```python
from build123d import *

# Parameters (mm, degrees)
F0_R     = 1.5
F1_DEPTH = 10
F2_DEPTH = 5
F3_DEPTH = 3


with BuildPart() as f1:
    # F0 (on Top) → F1 (new body)
    with BuildSketch(Plane.XY):
        Circle(F0_R)
    extrude(amount=F1_DEPTH)

    # F0 (on Top) → F2 (join)
    with BuildSketch(Plane.XY):
        Polygon((1.31021, 2.26935), (-1.31021, 2.26935), (-2.62042, 0), (-1.31021, -2.26935), (1.31021, -2.26935), (2.62042, 0), align=None)
        Circle(F0_R, mode=Mode.SUBTRACT)
    extrude(amount=F2_DEPTH)

    # F0 (on Top) → F3 (cut)
    with BuildSketch(Plane.XY):
        Circle(F0_R)
    extrude(amount=F3_DEPTH, mode=Mode.SUBTRACT)


solid = f1.part
```
For this review, take the finished solid that the model builds, in its own axes (mm). A direction names the side the tool comes from. Give positions to 0.01 mm unless a question says otherwise; leave off trailing zeros. Write each loop counter-clockwise with the first axis right and the second up, starting at its lowest first coordinate (ties: lowest second). Pieces come first, ordered by that corner, then holes.
Item 1: The part is to be moulded in two halves that separate along Y. For faces 3 (the face through (0, 2, 0)), 4 (the face through (0, 0, 3)), 5 (the face through (1.974, 1.119, 2.465)), 6 (the face through (-1.5, 0.07, 1.48)), say which applies: +Y half, -Y half, draft (parallel to the pull), parting line (faces both ways), or undercut.
Item 2: Wall thickness on probe 1 along Y at (x, z) = (0, 1.45); probe 2 along Z at (x, y) = (-0.5, 0.45); probe 3 along X at (y, z) = (-0.55, 2.5): over which ranges is each line inside the solid? List them lowest first.
Item 3: Take a section at B-B (x = 0). Give the boundary of the cut face in (y, z), and give its area (3 significant figures).
Item 4: Take a section at D-D (y = 0.15). Give the boundary of the cut face in (x, z), and give its area (3 significant figures).
Item 5: Take a section at A-A (z = 2). Give the boundary of the cut face in (x, y), and give its area (3 significant figures).
Item 6: Take a section at C-C (z = 4.75). Give the boundary of the cut face in (x, y), and give its area (3 significant figures).
Item 7: Insertion check: P1, Ø1.5, axis at y = -1, z = 6.5, coming from the -X side. The pin has a flat end and moves straight along its axis. Give the tip position at first contact, or say it passes through.
Item 8: Machinability: for faces 1 (the face through (0, -2.269, 2)), 2 (the face through (0, 2, 5)), which of the approach directions +Z, -Z, +X, -X, +Y, -Y give a long, thin tool a straight path to every point of the face, cutting with its end or side? Answer none if there is none.
Established:
1. face 3: draft
1. face 4: undercut
1. face 5: +Y half
1. face 6: undercut
2. probe 1: y = -2.27 to -1.5, 1.5 to 2.27
2. probe 2: z = 3 to 10
2. probe 3: x = -2.3 to -1.4, 1.4 to 2.3
3. outline: (-2.27, 0) - (-1.5, 0) - (-1.5, 3) - (1.5, 3) - (1.5, 0) - (2.27, 0) - (2.27, 5) - (1.5, 5) - (1.5, 10) - (-1.5, 10) - (-1.5, 5) - (-2.27, 5) - close
3. area: 28.7 mm2
4. outline: (-2.53, 0) - (-1.49, 0) - (-1.49, 3) - (1.49, 3) - (1.49, 0) - (2.53, 0) - (2.53, 5) - (1.49, 5) - (1.49, 10) - (-1.49, 10) - (-1.49, 5) - (-2.53, 5) - close
4. area: 31.3 mm2
5. outline: (-2.62, 0) - (-1.31, -2.27) - (1.31, -2.27) - (2.62, 0) - (1.31, 2.27) - (-1.31, 2.27) - close; hole circle Ø3 at (0, 0)
5. area: 10.8 mm2
6. outline: (-2.62, 0) - (-1.31, -2.27) - (1.31, -2.27) - (2.62, 0) - (1.31, 2.27) - (-1.31, 2.27) - close
6. area: 17.8 mm2
7. P1: stops at x = -1.48
8. face 1: +Z, -Z, +X, -X, -Y
8. face 2: +Z
